Input: part model. Units: mm. Frame: model coordinates. A direction names the side the tool comes from. Coordinates: 2 decimals unless noted, no trailing zeros. Order: outer loops, then holes, each group sorted by start corner. A loop starts at its lowest first (then second) coordinate and runs counter-clockwise, first axis right, second up. Notation, with made-up numbers: (50, 22) -> (82, 22) arc R15 cw to (82, 38) -> close; hole circle Ø7 at (-34, 2). An arc over 180 degrees is marked (long way). Use CSV: the item, a comma, the result in double quotes. Start each with the question number.
Autodesk Inventor part; units mm, degrees
ref_plane "YZ Plane" through (0, 0, 0) normal (1, 0, 0) x (0, 1, 0)
ref_plane "XZ Plane" through (0, 0, 0) normal (0, 1, 0) x (-1, 0, 0)
ref_plane "XY Plane" through (0, 0, 0) normal (0, 0, 1) x (1, 0, 0)
sketch "Sketch1" plane through (0, 0, 0) normal (0, 1, 0) x (-1, 0, 0)
  line L0 (0, 0) -> (50.8, 0)
  line L1 (50.8, 0) -> (50.8, -101.6)
  line L2 (50.8, -101.6) -> (0, -101.6)
  line L3 (0, -101.6) -> (0, 0)
  dimension "d0" = 50.8
  dimension "d1" = 101.6
extrude "Extrusion1" add sketch "Sketch1" along normal blind 914.4
sketch "Sketch2" plane through (-50.8, 0, 0) normal (0, 0, 1) x (1, 0, 0)
  line L0 (0, 0) -> (0, 914.4)
  line L1 (0, 914.4) -> (508, 914.4)
  line L2 (508, 914.4) -> (508, 533.4)
  line L3 (508, 533.4) -> (0, 533.4)
  line L4 (0, 533.4) -> (0, 914.4)
  point P0 (50.8, 0)
  dimension "d4" = 508
  dimension "d5" = 381
extrude "Extrusion2" add sketch "Sketch2" along normal blind 12.7
sketch "Sketch3" plane through (0, 0, -101.6) normal (0, 0, -1) x (-1, 0, 0)
  line L0 (0, 533.4) -> (0, 914.4)
  line L1 (0, 914.4) -> (-457.2, 914.4)
  line L2 (-457.2, 914.4) -> (-457.2, 533.4)
  line L3 (-457.2, 533.4) -> (0, 533.4)
  line L4 (-457.2, 914.4) -> (50.8, 914.4)
  line L5 (50.8, 914.4) -> (50.8, 533.4)
  line L6 (50.8, 533.4) -> (-457.2, 533.4)
  line L7 (-457.2, 533.4) -> (-457.2, 914.4)
  point P0 (0, 0)
extrude "Extrusion3" add sketch "Sketch3" along normal blind 12.7
sketch "Sketch4" plane through (0, 0, -101.6) normal (0, 0, 1) x (1, 0, 0)
  line L0 (457.2, 533.4) -> (0, 533.4)
  line L1 (457.2, 533.4) -> (406.4, 533.4)
  line L2 (406.4, 533.4) -> (406.4, 647.7)
  line L3 (406.4, 647.7) -> (457.2, 647.7)
  line L4 (457.2, 647.7) -> (457.2, 533.4)
  line L5 (406.4, 647.7) -> (457.2, 647.7)
  line L6 (457.2, 647.7) -> (457.2, 76.2)
  line L7 (457.2, 76.2) -> (406.4, 76.2)
  line L8 (406.4, 76.2) -> (406.4, 647.7)
  line L9 (457.2, 914.4) -> (-50.8, 914.4)
  point P0 (0, 0)
  dimension "d10" = 50.8
  dimension "d11" = 114.3
  dimension "d12" = 838.2
extrude "Extrusion4" add sketch "Sketch4" along normal up to surface (101.6 mm away)
sketch "Sketch5" plane through (0, 0, -101.6) normal (0, 0, 1) x (1, 0, 0)
  circle A0 centre (38.1, 889) radius 6.35
  circle A1 centre (292.1, 647.7) radius 6.35
  line L0 (-50.8, 914.4) -> (-50.8, 533.4)
  line L1 (457.2, 914.4) -> (-50.8, 914.4)
  line L2 (457.2, 533.4) -> (457.2, 914.4)
  line L3 (-50.8, 533.4) -> (457.2, 533.4)
  point P0 (0, 0)
  dimension "d15" = 12.7
  dimension "d16" = 12.7
  dimension "d17" = 88.9
  dimension "d18" = 25.4
  dimension "d20" = 165.1
  dimension "d21" = 114.3
extrude "Extrusion5" add sketch "Sketch5" along normal up to surface (101.6 mm away) contours A0 | A1
sketch "Sketch6" plane through (0, 0, -101.6) normal (0, 0, 1) x (1, 0, 0)
  line L0 (457.2, 914.4) -> (457.2, 647.7)
  line L1 (457.2, 863.6) -> (406.2091, 790.7774)
  line L2 (457.2, 863.6) -> (546.1, 863.6) construction
  line L3 (406.2091, 790.7774) -> (364.5961, 819.9151)
  line L4 (364.5961, 819.9151) -> (415.5871, 892.7377)
  line L5 (415.5871, 892.7377) -> (457.2, 863.6)
  line L6 (457.2, 914.4) -> (0, 914.4)
  point P0 (0, 0)
  dimension "d24" = 88.9
  dimension "d25" = 125
  dimension "d26" = 50.8
  dimension "d27" = 50.8
extrude "Extrusion6" add sketch "Sketch6" along normal up to surface (101.6 mm away)
properties part number "PBotCatapultShell"
1. Access query for faces 5 (the face through (389.735, 855.817, -51.511)), 6 (the face through (431, 647.7, -52)), 7 (the face through (432, 76.2, -52)), 8 (the face through (431, 308, 0)), 9 (the face through (-26, 263, -101.6)). Directions: +Z, -Z, +X, -X, +Y, -Y. A direction counts if a zero-diameter tool reaches every point of the face in a straight line with its end or side. Return the directions, or none.
2. Section B-B on x = 311.5. Return loops of the section in (y, z), then the cut area to 3 significant figures.
3. Contact query for flat-ended pins moving along their axis: P1, Ø6, axis at x = 401.5, z = -15.5, coming from the -Y side; P2, Ø15, axis at x = 441, y = 321.5, coming from the -Z side; P3, Ø4, axis at x = 328.5, z = -111, coming from the -Y side; P4, Ø2, axis at x = 300, z = -43, coming from the -Y side. Output: stop coordinate, or through.
4. Section A-A on z = -73.5. Return loops of the section in (x, y).
5. Material intervals for line 1 along X through (y, z) = (361, -47.5); line 2 along Z through (x, y) = (93.5, 591); line 3 along X through (y, z) = (654.5, -10), sorted ascending.
6. Pull-direction query (X, two-part tool) for faces 1 (the face through (457.2, 408, -52)), 2 (the face through (-25, 263, 0)), 3 (the face through (406.4, 358, -52)), 4 (the face through (-50.8, 451, -50)); classes: released by +X, released by -X, zero draft, split by the parting line, or undercut.
7. Section D-D on y = 577. Return loops of the section in (x, z).
8. Section C-C on y = 218.5. Return loops of the section in (x, z).
Values follow:
1,face 5,"+Y"
1,face 6,"+X"
1,face 7,"+Z, -Z, +X, -Y"
1,face 8,"+Z, +X, -X, -Y"
1,face 9,"-Z, +X, -X, -Y"
2,outline,"(533.4, -114.3) -> (914.4, -114.3) -> (914.4, -101.6) -> (533.4, -101.6) -> close; (533.4, 0) -> (914.4, 0) -> (914.4, 12.7) -> (533.4, 12.7) -> close"
2,area,"9,680 mm2"
3,P1,"stops at y = 791.97"
3,P2,"stops at z = -101.6"
3,P3,"stops at y = 533.4"
3,P4,"passes through"
4,outline,"(-50.8, 0) -> (0, 0) -> (0, 914.4) -> (-50.8, 914.4) -> close; circle Ø12.7 at (38.1, 889); circle Ø12.7 at (292.1, 647.7); (364.6, 819.92) -> (406.21, 790.78) -> (457.2, 863.6) -> (415.59, 892.74) -> close; (406.4, 76.2) -> (457.2, 76.2) -> (457.2, 647.7) -> (406.4, 647.7) -> close"
5,line 1,"x = -50.8 to 0, 406.4 to 457.2"
5,line 2,"z = -114.3 to -101.6, 0 to 12.7"
5,line 3,"x = -50.8 to 0"
6,face 1,"released by +X"
6,face 2,"zero draft"
6,face 3,"undercut"
6,face 4,"released by -X"
7,outline,"(-50.8, -114.3) -> (457.2, -114.3) -> (457.2, 12.7) -> (-50.8, 12.7) -> close; hole (0, -101.6) -> (406.4, -101.6) -> (406.4, 0) -> (0, 0) -> close"
8,outline,"(-50.8, -101.6) -> (0, -101.6) -> (0, 0) -> (-50.8, 0) -> close; (406.4, -101.6) -> (457.2, -101.6) -> (457.2, 0) -> (406.4, 0) -> close"
